Geometry check sheet. Reference: the model listing, model coordinates, mm. Round coordinates to 2 decimals unless told otherwise and drop trailing zeros. Write each loop counter-clockwise with the first axis right and the second up, starting at its lowest first coordinate (ties: lowest second). Pieces come first, ordered by that corner, then holes. Notation, with made-up numbers: (43.25, 3) - (54.25, 3) arc R24 ccw to (54.25, 41) - close; hole circle Ø2 at (20, 70). An arc over 180 degrees is marked (long way). One line per question, with ' | ' between items. Start each with the question number.
from build123d import *
from OCP.BRepFilletAPI import BRepFilletAPI_MakeChamfer

# Parameters (mm, degrees)
SKETCH1_R           = 3.175
SKETCH1_R_2         = 1.2999974
BOSS_EXTRUDE1_DEPTH = 14.26875
DRAFT2_ANGLE        = -2
CHAMFER1_SIZE       = 0.508
CHAMFER1_SIZE2      = 0.526702505


with BuildPart() as part:
    # Sketch1 → Boss-Extrude1 (new body)
    with BuildSketch(Plane.XY):
        with Locations(Location((0, 6.009690382, 0), (0, 0, 270))):
            Circle(SKETCH1_R)
        with Locations(Location((0, 6.009690382, 0), (0, 0, 270))):
            Circle(SKETCH1_R_2, mode=Mode.SUBTRACT)
    extrude(amount=BOSS_EXTRUDE1_DEPTH)

    # Draft2
    draft2_faces = [part.faces().sort_by_distance(p)[0] for p in [
        (0, 7.309687782, 7.134375),
    ]]
    draft(draft2_faces, Plane(origin=(0, 6.009690382, 0), x_dir=(-1, 0, 0), z_dir=(0, 0, -1)), DRAFT2_ANGLE)

    # Chamfer1: one chamfer whose edges measure the first distance from different faces: ONE call of the kernel's chamfer builder (chamfer() names one face for all edges)
    chamfer1_edges_1 = [part.edges().sort_by_distance(p)[0] for p in [
        (0, 9.184690382, 14.26875),
        (0, 9.184690382, 0),
    ]]
    chamfer1_edges_2 = [part.edges().sort_by_distance(p)[0] for p in [
        (0, 7.807963512, 14.26875),
    ]]
    chamfer1_side_2 = [part.faces().sort_by_distance(p)[0] for p in [
        (0, 9.094887821, 14.26875),
    ]]
    chamfer1 = BRepFilletAPI_MakeChamfer(part.part.solid().wrapped)
    for e in chamfer1_edges_1:
        chamfer1.Add(CHAMFER1_SIZE, e.wrapped)
    for e in chamfer1_edges_2:
        chamfer1.Add(CHAMFER1_SIZE, CHAMFER1_SIZE2, e.wrapped, chamfer1_side_2[0].wrapped)  # the first distance lies on this face
    add(Compound.cast(chamfer1.Shape()), mode=Mode.REPLACE)


solid = part.part
Q1. Section check A-A, the plane x = 0. Record the cut outline in (y, z), then the cut area to 3 significant figures.
Q2. Section check C-C, the plane z = 5.25. Record the cut outline in (x, y) (3 decimals), then the cut area to 3 significant figures.
Q3. Section check B-B, the plane z = 6.75. Record the cut outline in (x, y) (3 decimals).
Q4. Go/stop test with a flat-tipped pin: P1, Ø3, axis at x = 2.5, z = 8, coming from the +Y side. Record where the tip stops, or that it passes through.
Q5. Thickness scan on line 1 (X direction, y = 6.5, z = 6.75); line 2 (X direction, y = 5, z = 10.5); line 3 (Y direction, x = 1, z = 12.5). Record the ranges inside material, lowest first.
Q6. Draft check along X on faces 1 (the cylindrical face through (-1.93, 8.53, 7.04)), 2 (the conical face through (0.068, 7.545, 6.775)). Enter one of: pulls with the +X half, pulls with the -X half, needs draft (parallel to the pull), parting line crosses it, or undercut.
Result sheet:
1) outline: (2.83, 0.51) - (3.34, 0) - (4.71, 0) - (4.23, 13.74) - (3.7, 14.27) - (3.34, 14.27) - (2.83, 13.76) - close; (7.31, 0) - (8.68, 0) - (9.18, 0.51) - (9.18, 13.76) - (8.68, 14.27) - (8.32, 14.27) - (7.79, 13.74) - close | area: 45.6 mm²
2) outline: circle Ø6.35 at (0, 6.01); hole circle Ø2.967 at (0, 6.01) | area: 24.8 mm²
3) outline: circle Ø6.35 at (0, 6.01); hole circle Ø3.071 at (0, 6.01)
4) P1: y = 9.02
5) line 1: -3.14 to -1.46, 1.46 to 3.14 | line 2: -3.01 to -1.33, 1.33 to 3.01 | line 3: 3 to 4.59, 7.43 to 9.02
6) face 1: parting line crosses it | face 2: undercut
